Read the model definition and answer for the solid it produces. Units are mm, in the model's axes. A direction names the side the tool comes from. Coordinates: 2 decimals unless noted, no trailing zeros. Write each loop counter-clockwise with the first axis right and the second up, starting at its lowest first coordinate (ties: lowest second). Pieces come first, ordered by that corner, then holes.
(1) The part is cut by section A-A, the plane x = -10.5. Determine the outline of the cut face in (y, z).
(2) Given pin 1 (2 mm diameter, centred on y = -54, z = 88.5, fed in from +X); pin 2 (14.5 mm diameter, centred on y = -38.5, z = 10, fed in from -X); pin 3 (12 mm diameter, centred on y = -21.5, z = 52, fed in from +X), each flat-ended and moving along its own axis, determine where each tip first touches the part or whether it passes through.
(3) Straight lines are drawn through the part: line 1 along Z through (x, y) = (128.5, -31.5); line 2 along Y through (x, z) = (-7, 37.5); line 3 along Z through (x, y) = (28, -22.5). For each, find the intervals that lie inside material, in ascending order.
(4) Which of the six approach directions +Z, -Z, +X, -X, +Y, -Y give full straight-line access (tool end or side, diameter ignored) to faces 1 (the flat face through (76, -32, 19)), 2 (the flat face through (-20.644, -31.594, 41.756)), 3 (the cylindrical face through (28.22, -31.36, 111.11))?
(5) The part is cut by section B-B, the plane x = 59. Determine the outline of the cut face in (y, z), and give its area (3 significant figures).
(6) Determine the mould class of faces 4 (the flat face through (69, -32, 0)), 5 (the flat face through (68, -32, 3)), 6 (the flat face through (27, -61, 13)), 7 (the flat face through (140, -32, 9)) for opening direction X: pulls with the +X half, pulls with the -X half, needs draft (parallel to the pull), parting line crosses it, or undercut.
(7) The part is cut by section D-D, the plane z = 25.5. Determine the outline of the cut face in (x, y).
(8) The part is cut by section C-C, the plane y = -19.5. Determine the outline of the cut face in (x, z), and give its area (3 significant figures).
```python
from build123d import *

# Parameters (mm, degrees)
F2_DEPTH = 64
F4_DEPTH = 19
F5_T     = -3
F6_R     = 9.5
F7_DEPTH = 3


with BuildPart() as f2:
    # F1 (on Front) → F2 (new body)
    with BuildSketch(Plane.XZ):
        Polygon((0, 0), (140, 0), (140, 19), (10.9696551146, 19), (-19.0455173281, 70.9878036687), (64.0929214352, 118.9878036687), (54.5929214352, 135.4422863406), (-45, 77.9422863406), align=None)
    extrude(amount=F2_DEPTH)

    # F3 (on face) → F4 (cut, through all)
    with BuildSketch(Plane(origin=(-45, 0, 77.9422863406), x_dir=(0.8660254038, 0, 0.5), z_dir=(-0.5, 0, 0.8660254038))):
        with BuildLine():
            ThreePointArc((51, 0), (83, -32), (51, -64))
            Line((51, -64), (115, -64))
            Line((115, -64), (115, 0))
            Line((115, 0), (51, 0))
        make_face()
    extrude(amount=-F4_DEPTH, mode=Mode.SUBTRACT)

    # F5
    f5_openings = [f2.faces().sort_by_distance(p)[0] for p in [
        (-11.74342, -32, 97.142982),
    ]]
    offset(amount=F5_T, openings=f5_openings, kind=Kind.INTERSECTION)

    # F6 (on face) → F7 (cut, through all)
    with BuildSketch(Plane(origin=(-37, 0, 64.08587988), x_dir=(0.8660254038, 0, 0.5), z_dir=(-0.5, 0, 0.8660254038))):
        with Locations((51.0000000002, -32)):
            Circle(F6_R)
    extrude(amount=-F7_DEPTH, mode=Mode.SUBTRACT)


solid = f2.part
```
Computed:
1. outline: (-64, 18.19) - (0, 18.19) - (0, 56.19) - (-64, 56.19) - close; (-64, 75.92) - (0, 75.92) - (0, 97.86) - (-3, 97.86) - (-3, 79.39) - (-61, 79.39) - (-61, 97.86) - (-64, 97.86) - close; hole (-61, 24.19) - (-3, 24.19) - (-3, 50.19) - (-61, 50.19) - close
2. pin 1: stops at x = 13.02
2. pin 2: stops at x = -9.96
2. pin 3: stops at x = -4.62
3. line 1: z = 0 to 3, 16 to 19
3. line 2: y = -64 to -61, -3 to 0
3. line 3: z = 0 to 3, 16 to 19, 98.15 to 101.61, 108.3 to 114.62
4. face 1: +X, +Y, -Y
4. face 2: none
4. face 3: -X
5. outline: (-64, 0) - (0, 0) - (0, 19) - (-64, 19) - close; hole (-61, 3) - (-3, 3) - (-3, 16) - (-61, 16) - close
5. area: 462 mm2
6. face 4: needs draft
6. face 5: undercut
6. face 6: undercut
6. face 7: pulls with the +X half
7. outline: (-14.72, -64) - (7.22, -64) - (7.22, 0) - (-14.72, 0) - close; hole (-11.26, -61) - (3.75, -61) - (3.75, -3) - (-11.26, -3) - close
8. outline: (-45, 77.94) - (0, 0) - (140, 0) - (140, 19) - (10.97, 19) - (-19.05, 70.99) - (34.18, 101.72) - (24.68, 118.17) - (21.83, 116.53) - (29.83, 102.67) - (-23.14, 72.09) - (9.24, 16) - (137, 16) - (137, 3) - (1.73, 3) - (-42.4, 79.44) - close
8. area: 1,540 mm2
